Here's how the part is built. I have some questions about the finished solid (model axes, mm). Round coordinates to 2 decimals unless told otherwise and drop trailing zeros. Write each loop counter-clockwise with the first axis right and the second up, starting at its lowest first coordinate (ties: lowest second). Pieces come first, ordered by that corner, then holes. Notation, with made-up numbers: (-19, 73.5) -> (27, 73.5) arc R27 cw to (27, 109.5) -> close; hole circle Ø6 at (29.25, 41). An arc over 180 degrees is marked (long way). Answer in a Markdown table with one row per item.
from build123d import *

# Parameters (mm, degrees)
F0_W     = 96.524141
F0_H     = 35.803635
F1_DEPTH = 25.4
F2_R     = 12.877415
F3_SIZE  = 12.7


with BuildPart() as f1:
    # F0 (on Top) → F1 (new body)
    with BuildSketch(Plane.XY):
        with Locations((-13.090502, -17.901817)):
            Rectangle(F0_W, F0_H)
    extrude(amount=F1_DEPTH)

    # F2
    f2_edges = [f1.edges().sort_by_distance(p)[0] for p in [
        (-13.090502, -35.803635, 25.4),
    ]]
    fillet(f2_edges, radius=F2_R)

    # F3
    f3_edges = [f1.edges().sort_by_distance(p)[0] for p in [
        (-13.090502, 0, 25.4),
    ]]
    chamfer(f3_edges, length=F3_SIZE)


solid = f1.part
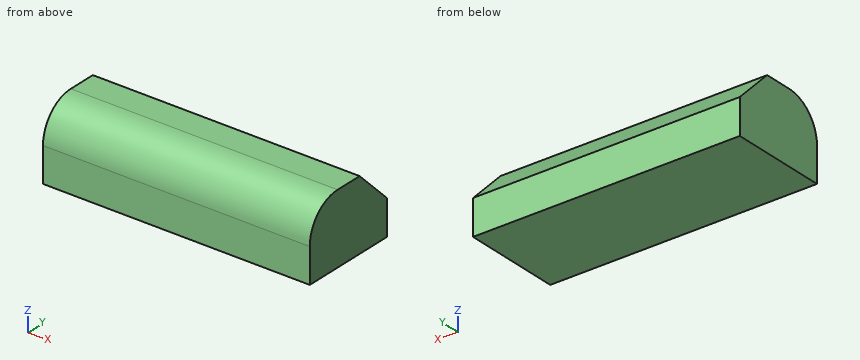
1) I need wall thicknesses on line 1 (Z direction, x = -13, y = -28.5); line 2 (Y direction, x = -27, z = 21.75); line 3 (Y direction, x = 14.5, z = 24.25). Which ranges of each line are inside material? Lowest first, please. Write a range as [from, to].
Response:
| item | result |
|---|---|
| line 1 | z = [0, 24.13] |
| line 2 | y = [-31.91, -9.05] |
| line 3 | y = [-28.25, -11.55] |
2) I want a section at C-C, the plane y = -4. List the corners of the cut face in (x, z) for me, and give its area (3 significant figures).
Response:
| item | result |
|---|---|
| outline | (-61.35, 0) -> (35.17, 0) -> (35.17, 16.7) -> (-61.35, 16.7) -> close |
| area | 1,610 mm^2 |
3) I want a section at B-B, the plane z = 14.25. List the corners of the cut face in (x, y) for me.
Response:
| item | result |
|---|---|
| outline | (-61.35, -35.69) -> (35.17, -35.69) -> (35.17, -1.55) -> (-61.35, -1.55) -> close |
4) I want a section at A-A, the plane x = 29. List the corners of the cut face in (y, z) for me.
Response:
| item | result |
|---|---|
| outline | (-35.8, 0) -> (0, 0) -> (0, 12.7) -> (-12.7, 25.4) -> (-22.93, 25.4) arc R12.88 ccw to (-35.8, 12.52) -> close |
